from build123d import *

# Parameters (mm, degrees)
F0_R     = 10
F0_R_2   = 20
F0_R_3   = 2.5
F1_DEPTH = 7.5


with BuildPart() as f1:
    # F0 (on Front) → F1 (new body, symmetric)
    with BuildSketch(Plane.XZ):
        with BuildLine():
            ThreePointArc((-276.017555, -20.660086), (-266.304674, -35.067994), (-250.261343, -41.741776))
            Line((-250.261343, -41.741776), (207.324587, -88.806799))
            ThreePointArc((207.324587, -88.806799), (253.185254, -84.115685), (293.400793, -61.578656))
            Line((293.400793, -61.578656), (709.601084, 299.95794))
            ThreePointArc((709.601084, 299.95794), (721.746277, 314.620589), (723.932064, 333.534112))
            Line((723.932064, 333.534112), (701.375468, 462.389844))
            ThreePointArc((701.375468, 462.389844), (683.514294, 486.942452), (654.636412, 496.31902))
            Line((654.636412, 496.31902), (-79.706343, 496.31902))
            Line((-79.706343, 496.31902), (-79.706343, 481.31902))
            Line((-79.706343, 481.31902), (-94.706343, 481.31902))
            Line((-94.706343, 481.31902), (-94.706343, 496.31902))
            Line((-94.706343, 496.31902), (-134.706343, 496.31902))
            Line((-134.706343, 496.31902), (-134.706343, 481.31902))
            Line((-134.706343, 481.31902), (-149.706343, 481.31902))
            Line((-149.706343, 481.31902), (-149.706343, 496.31902))
            Line((-149.706343, 496.31902), (-189.706343, 496.31902))
            Line((-189.706343, 496.31902), (-189.706343, 481.31902))
            Line((-189.706343, 481.31902), (-204.706343, 481.31902))
            Line((-204.706343, 481.31902), (-204.706343, 496.31902))
            Line((-204.706343, 496.31902), (-244.706343, 496.31902))
            Line((-244.706343, 496.31902), (-244.706343, 481.31902))
            Line((-244.706343, 481.31902), (-259.706343, 481.31902))
            Line((-259.706343, 481.31902), (-259.706343, 496.31902))
            Line((-259.706343, 496.31902), (-299.706343, 496.31902))
            Line((-299.706343, 496.31902), (-299.706343, 481.31902))
            Line((-299.706343, 481.31902), (-314.706343, 481.31902))
            Line((-314.706343, 481.31902), (-314.706343, 496.31902))
            Line((-314.706343, 496.31902), (-354.706343, 496.31902))
            Line((-354.706343, 496.31902), (-354.706343, 481.31902))
            Line((-354.706343, 481.31902), (-369.706343, 481.31902))
            Line((-369.706343, 481.31902), (-369.706343, 496.31902))
            Line((-369.706343, 496.31902), (-395.363588, 496.31902))
            ThreePointArc((-395.363588, 496.31902), (-419.90474, 483.912815), (-424.465387, 456.794876))
            Line((-424.465387, 456.794876), (-276.017555, -20.660086))
        make_face()
        with Locations((-232.248772, -13.546013)):
            Circle(F0_R, mode=Mode.SUBTRACT)
        with BuildLine():
            Line((-205.025903, 54.145206), (-294.760891, 342.761177))
            ThreePointArc((-294.760891, 342.761177), (-288.05875, 379.583252), (-254.581922, 396.31902))
            Line((-254.581922, 396.31902), (152.180821, 396.31902))
            add(Edge.make_bspline(
                [(152.180821, 396.31902), (202.900278, 395.792604), (182.017022, 350.09414), (234.05233, 346.31902)],
                knots=[0, 0, 0, 0, 95.931976, 95.931976, 95.931976, 95.931976], degree=3))
            Line((234.05233, 346.31902), (511.96432, 346.31902))
            ThreePointArc((511.96432, 346.31902), (551.787832, 318.687201), (539.843978, 271.71089))
            Line((539.843978, 271.71089), (239.642025, 10.937424))
            ThreePointArc((239.642025, 10.937424), (224.102433, 2.114935), (206.358638, 0))
            Line((206.358638, 0), (-175.751697, 30.723296))
            ThreePointArc((-175.751697, 30.723296), (-193.976565, 37.950032), (-205.025903, 54.145206))
        make_face(mode=Mode.SUBTRACT)
        with Locations((230.366445, -43.535308)):
            Circle(F0_R_2, mode=Mode.SUBTRACT)
        with Locations((-415.037585, 459.662208)):
            Circle(F0_R_3, mode=Mode.SUBTRACT)
        with Locations((-414.954704, 476.152515)):
            Circle(F0_R_3, mode=Mode.SUBTRACT)
        with Locations((-404.460467, 487.250969)):
            Circle(F0_R_3, mode=Mode.SUBTRACT)
        with BuildLine():
            ThreePointArc((-348.862556, 424.598233), (-363.862556, 439.598233), (-348.862556, 454.598233))
            Line((-348.862556, 454.598233), (-78.862556, 454.598233))
            ThreePointArc((-78.862556, 454.598233), (-63.862556, 439.598233), (-78.862556, 424.598233))
            Line((-78.862556, 424.598233), (-348.862556, 424.598233))
        make_face(mode=Mode.SUBTRACT)
        with Locations((677.034383, 471.78393)):
            Circle(F0_R_3, mode=Mode.SUBTRACT)
    extrude(amount=F1_DEPTH, both=True)


solid = f1.part
Part model, mm, in its own coordinate system. A direction names the side the tool comes from. Coordinates: 2 decimals unless noted, no trailing zeros. Loops run counter-clockwise (first coordinate to the right, second up) from the corner with the lowest first, then second, coordinate; pieces in that order, holes last. Notation, with made-up numbers: M -12.5,48 L 22.5,48 A16 ccw 22.5,61 Z; hole C 18.5,46 d10. An arc over 180 degrees is marked long. Use a Markdown table: item, result. Add a question column.
Q1. Cut at B-B (z = 100.5). Write the cut outline in (x, y).
Q2. Cut at C-C (y = 3.75). Give the number of separate pieces and of enclosed holes in the cut face, and give its area (3 significant figures).
Q3. Which spindle directions (+Z, -Z, +X, -X, +Y, -Y) get a long thin tool onto all of the face, cutting with end or side? Do faces 1 (the cylindrical face through (-266.495, -0.105, -34.911)), 2 (the cylindrical face through (-193.76, -0.11, 37.78)). Say none if no direction does.
Q4. Mould opens along X. For faces 3 (the flat face through (-249.265, -0.105, 196.433)), 4 (the flat face through (712.81, -0.11, 397.06)), 5 (the cylindrical face through (-419.67, -0.11, 484.23)) say: +X half, -X half, draft (parallel to the pull), parting line (faces both ways), or undercut.
Q5. Probe L1, parallel to Z at x = -129, y = -7; L2, parallel to Z at x = -155.5, y = -5.25; L3, parallel to X at y = -3.5, z = 267. List the from-to ranges inside material, lowest first.
Q6. Pin check, flat tips, straight feed: P1, Ø6, axis at x = 542, y = 1, coming from the -Z side; P2, Ø2, axis at y = -1.5, z = 316, coming from the +X side; P3, Ø1, axis at y = 1.5, z = 176.5, coming from the -X side; P4, Ø4, axis at x = -415.04, z = 459.66, coming from the +Y side. Stop position of each tip, or through.
Q7. Cut at A-A (x = 381). Write the cut outline in (y, z), and give its area (3 significant figures).
Worked out:
| question | item | result |
|---|---|---|
| 1 | outline | M -313.69,-7.5 L -219.44,-7.5 L -219.44,7.5 L -313.69,7.5 Z; M 342.75,-7.5 L 479.99,-7.5 L 479.99,7.5 L 342.75,7.5 Z |
| 2 | separate pieces | 1 |
| 2 | enclosed holes | 8 |
| 2 | area | 260,000 mm2 |
| 3 | face 1 | -Z, -X, +Y, -Y |
| 3 | face 2 | +Y, -Y |
| 4 | face 3 | undercut |
| 4 | face 4 | +X half |
| 4 | face 5 | -X half |
| 5 | L1 | z = -54.21 to 26.96, 396.32 to 424.6, 454.6 to 496.32 |
| 5 | L2 | z = -51.49 to 29.09, 396.32 to 424.6, 454.6 to 496.32 |
| 5 | L3 | x = -365.46 to -271.21, 534.42 to 671.66 |
| 6 | P1 | stops at z = 151.76 |
| 6 | P2 | stops at x = 722.66 |
| 6 | P3 | stops at x = -337.47 |
| 6 | P4 | passes through |
| 7 | outline | M -7.5,14.52 L 7.5,14.52 L 7.5,133.73 L -7.5,133.73 Z; M -7.5,346.32 L 7.5,346.32 L 7.5,496.32 L -7.5,496.32 Z |
| 7 | area | 4,040 mm2 |
